Design review of the part built by this model. Coordinates are the model's own, in mm. Face numbers are marked on the shaded views. A direction names the side the tool comes from. Round coordinates to 2 decimals unless told otherwise and drop trailing zeros. Write each loop counter-clockwise with the first axis right and the second up, starting at its lowest first coordinate (ties: lowest second). Pieces come first, ordered by that corner, then holes. Notation, with made-up numbers: M -5.5,-38 L 46.5,-38 A27 cw 46.5,-7 Z; hole C 3.25,27.25 d9. An arc over 180 degrees is marked long. One line per question, with ' | ' between items. Start each with the question number.
Item 1: For L1, parallel to Y at x = 10.5, z = 9.1; L2, parallel to Y at x = 5.25, z = 4.5; L3, parallel to Y at x = 10.5, z = 6, list the stretches that pass through material, from the lowest coordinate up.
Item 2: Add section D-D, the plane y = 18.05. State the section outline as (x, z) points.
Item 3: Add section C-C, the plane z = 1. State the section outline as (x, y) points, and give its area (3 significant figures).
Item 4: Insertion check: pin 1 Ø2 at (y, z) = (3, 9) entering from -X. The pin has a flat end and moves straight along its axis. Give the tip position at first contact, or say it passes through.
Item 5: Add section A-A, the plane y = 11.05. State the section outline as (x, z) points.
Item 6: Add section B-B, the plane x = 15.75. State the section outline as (y, z) points, and give its area (3 significant figures).
Item 7: Machinability: for the marked faces 4 and 5, which of the approach directions +Z, -Z, +X, -X, +Y, -Y give a long, thin tool a straight path to every point of the face, cutting with its end or side? Answer none if there is none.
Item 8: Draft analysis for pull direction Y (two halves, no side actions). For the marked faces 1, 2 and 3, state which applies: released by +Y, released by -Y, zero draft, split by the parting line, or undercut.
```python
from build123d import *

# Parameters (mm, degrees)
F0_W     = 21
F0_H     = 22.1
F1_DEPTH = 11
F2_R     = 1.75
F3_DEPTH = 25
F2_R_2   = 3.35
F2_R_3   = 3.3
F4_DEPTH = 3.5
F6_R     = 5
F5_R     = 5
F7_DEPTH = 25


with BuildPart() as f1:
    # F0 (on Top) → F1 (new body)
    with BuildSketch(Plane.XY):
        with Locations((10.5, 11.05)):
            Rectangle(F0_W, F0_H)
    extrude(amount=F1_DEPTH)

    # F2 (on face) → F3 (cut)
    with BuildSketch(Plane.XY.offset(11)):
        with Locations((10.5, 18.05)):
            Circle(F2_R)
        with Locations((10.5, 4.05)):
            Circle(F2_R)
    extrude(amount=-F3_DEPTH, mode=Mode.SUBTRACT)

    # F2 (on face) → F4 (cut)
    with BuildSketch(Plane.XY.offset(11)):
        with Locations((10.5, 18.05)):
            Circle(F2_R_2)
        with Locations((10.5, 18.05)):
            Circle(F2_R, mode=Mode.SUBTRACT)
        with Locations((10.5, 4.05)):
            Circle(F2_R_3)
        with Locations((10.5, 4.05)):
            Circle(F2_R, mode=Mode.SUBTRACT)
    extrude(amount=-F4_DEPTH, mode=Mode.SUBTRACT)

    # F6
    f6_edges = [f1.edges().sort_by_distance(p)[0] for p in [
        (0, 22.1, 5.5),
        (0, 0, 5.5),
    ]]
    fillet(f6_edges, radius=F6_R)

    # F5 (on face) → F7 (cut)
    with BuildSketch(Plane.XY.offset(11)):
        with Locations((5.25, 11.05)):
            Circle(F5_R)
        with Locations((15.75, 11.05)):
            Circle(F5_R)
    extrude(amount=-F7_DEPTH, mode=Mode.SUBTRACT)


solid = f1.part
```
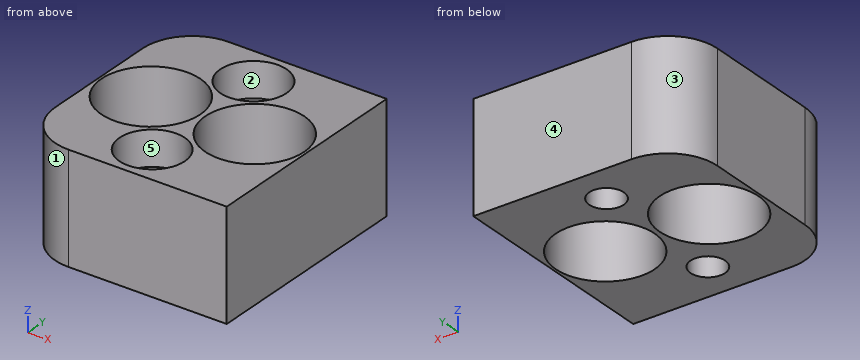
Computed values:
1) L1: y = 0 to 0.75, 7.35 to 14.7, 21.4 to 22.1 | L2: y = 0 to 6.05, 16.05 to 22.1 | L3: y = 0 to 2.3, 5.8 to 16.3, 19.8 to 22.1
2) outline: M 0.09,0 L 8.75,0 L 8.75,7.5 L 7.15,7.5 L 7.15,11 L 0.09,11 Z; M 12.25,0 L 21,0 L 21,11 L 13.85,11 L 13.85,7.5 L 12.25,7.5 Z
3) outline: M 0,5 A5 ccw 5,0 L 21,0 L 21,22.1 L 5,22.1 A5 ccw 0,17.1 Z; hole C 5.25,11.05 d10; hole C 10.5,4.05 d3.5; hole C 10.5,18.05 d3.5; hole C 15.75,11.05 d10 | area: 277 mm^2
4) pin 1: stops at x = 0.1
5) outline: M 0,0 L 0.25,0 L 0.25,11 L 0,11 Z; M 10.25,0 L 10.75,0 L 10.75,11 L 10.25,11 Z; M 20.75,0 L 21,0 L 21,11 L 20.75,11 Z
6) outline: M 0,0 L 6.05,0 L 6.05,11 L 0,11 Z; M 16.05,0 L 22.1,0 L 22.1,11 L 16.05,11 Z | area: 133 mm^2
7) face 4: +Z, -Z, +X, -X, +Y | face 5: +Z
8) face 1: released by -Y | face 2: undercut | face 3: released by +Y
